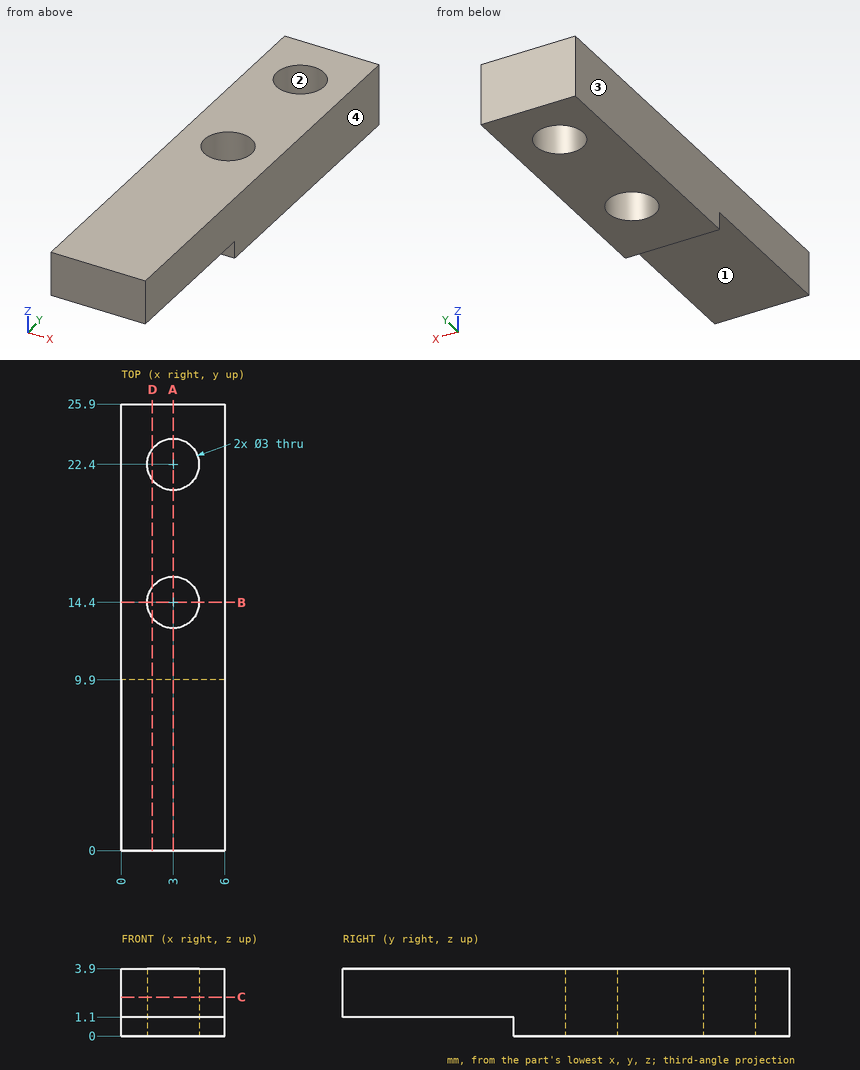
Can you work these out from the drawing? Everything is in mm from the part's minimum corner. Round coordinates to 2 decimals unless told otherwise and drop trailing zeros. Loops run counter-clockwise (first coordinate to the right, second up) from the corner with the lowest first, then second, coordinate; pieces in that order, holes last. Notation, with made-up numbers: (-16.75, -34.5) -> (14.25, -34.5) arc R20 cw to (14.25, -7.5) -> close; hole circle Ø4 at (41.25, 50.5). An arc over 180 degrees is marked (long way). One line per question, with ' | ' between items.
(1) If we section it at B-B on y = 14.4: List the corners of the cut face in (x, z) for me.
Model answer:
outline: (0, 0) -> (1.5, 0) -> (1.5, 3.9) -> (0, 3.9) -> close; (4.5, 0) -> (6, 0) -> (6, 3.9) -> (4.5, 3.9) -> close
(2) If we section it at C-C on z = 2.25: List the corners of the cut face in (x, y) for me.
Model answer:
outline: (0, 0) -> (6, 0) -> (6, 25.9) -> (0, 25.9) -> close; hole circle Ø3 at (3, 14.4); hole circle Ø3 at (3, 22.4)
(3) If we section it at D-D on x = 1.8: List the corners of the cut face in (y, z) for me.
Model answer:
outline: (0, 1.1) -> (9.9, 1.1) -> (9.9, 0) -> (13.5, 0) -> (13.5, 3.9) -> (0, 3.9) -> close; (15.3, 0) -> (21.5, 0) -> (21.5, 3.9) -> (15.3, 3.9) -> close; (23.3, 0) -> (25.9, 0) -> (25.9, 3.9) -> (23.3, 3.9) -> close
(4) If we section it at A-A on x = 3: List the corners of the cut face in (y, z) for me.
Model answer:
outline: (0, 1.1) -> (9.9, 1.1) -> (9.9, 0) -> (12.9, 0) -> (12.9, 3.9) -> (0, 3.9) -> close; (15.9, 0) -> (20.9, 0) -> (20.9, 3.9) -> (15.9, 3.9) -> close; (23.9, 0) -> (25.9, 0) -> (25.9, 3.9) -> (23.9, 3.9) -> close
(5) Thinking about a two-plate mould opening in X: for the marked faces 1, 2, 3 and 4, which applies, released by +X, released by -X, zero draft, split by the parting line, or undercut?
Model answer:
face 1: zero draft | face 2: undercut | face 3: released by -X | face 4: released by +X
(6) If I drill on probe 1 along Y at (x, z) = (3, 1.9); probe 2 along Y at (x, z) = (3, 0.95); probe 3 along X at (y, z) = (14.4, 1), over which ranges is the centre line in solid material (lowest first)?
Model answer:
probe 1: y = 0 to 12.9, 15.9 to 20.9, 23.9 to 25.9 | probe 2: y = 9.9 to 12.9, 15.9 to 20.9, 23.9 to 25.9 | probe 3: x = 0 to 1.5, 4.5 to 6
